CAD build for the part. Positions are in the model's coordinates, mm. A direction names the side the tool comes from. Round coordinates to 2 decimals unless told otherwise and drop trailing zeros. Order: outer loops, then holes, each group sorted by start corner. A loop starts at its lowest first (then second) coordinate and runs counter-clockwise, first axis right, second up. Notation, with made-up numbers: M -13,82.25 L -1,82.25 A14 ccw -1,102.25 Z; hole C 35,17.25 d9. An arc over 180 degrees is marked long. Answer as a JSON object with one key per item and string values.
```python
from build123d import *

# Parameters (mm, degrees)
BOSS_EXTRUDE1_DEPTH       = 138
CUT_EXTRUDE1_DEPTH        = 187.721718073
F_6_0MM_DOWEL_HOLE1_D     = 6
F_6_0MM_DOWEL_HOLE1_DEPTH = 28.197418143
F_6_0MM_DOWEL_HOLE1_TIP   = 1.802581857
M6X1_0_TAPPED_HOLE1_D     = 5
M6X1_0_TAPPED_HOLE1_DEPTH = 21.497848452
M6X1_0_TAPPED_HOLE1_TIP   = 1.502151548
CHAMFER1_SIZE             = 2


with BuildPart() as part:
    # Sketch1 → Boss-Extrude1 (new body)
    with BuildSketch(Plane.XY):
        Polygon((-125, 202.5), (-125, 197.5), (-125, 193), (0, 193), (0, 207), (-125, 207), align=None)
    extrude(amount=BOSS_EXTRUDE1_DEPTH)

    # Sketch3 → Cut-Extrude1 (cut, through all)
    with BuildSketch(Plane(origin=(0, 207, 0), x_dir=(1, 0, 0), z_dir=(0, 1, 0))):
        with BuildLine():
            Line((-105, -30), (-105, -108))
            ThreePointArc((-105, -108), (-102.071067812, -115.071067812), (-95, -118))
            Line((-95, -118), (-30, -118))
            ThreePointArc((-30, -118), (-22.928932188, -115.071067812), (-20, -108))
            Line((-20, -108), (-20, -35.297163281))
            ThreePointArc((-20, -35.297163281), (-18.9403759, -30.817243777), (-15.986064246, -27.286730407))
            ThreePointArc((-15.986064246, -27.286730407), (-14.821532054, -21.896326846), (-20, -20))
            Line((-20, -20), (-95, -20))
            ThreePointArc((-95, -20), (-102.071067812, -22.928932188), (-105, -30))
        make_face()
    extrude(amount=-CUT_EXTRUDE1_DEPTH, mode=Mode.SUBTRACT)

    # Ø6.0mm Dowel Hole1
    with Locations(Plane.XY.offset(20)):
        with Locations((-25, 200), (-55, 200), (-85, 200)):
            Hole(F_6_0MM_DOWEL_HOLE1_D / 2, depth=F_6_0MM_DOWEL_HOLE1_DEPTH)
            with Locations((0, 0, -(F_6_0MM_DOWEL_HOLE1_DEPTH + F_6_0MM_DOWEL_HOLE1_TIP / 2))):  # 118° drill point
                Cone(0, F_6_0MM_DOWEL_HOLE1_D / 2, F_6_0MM_DOWEL_HOLE1_TIP, mode=Mode.SUBTRACT)

    # M6x1.0 Tapped Hole1
    with Locations(Plane.XY.offset(138)):
        with Locations((-95, 200), (-30, 200)):
            Hole(M6X1_0_TAPPED_HOLE1_D / 2, depth=M6X1_0_TAPPED_HOLE1_DEPTH)
            with Locations((0, 0, -(M6X1_0_TAPPED_HOLE1_DEPTH + M6X1_0_TAPPED_HOLE1_TIP / 2))):  # 118° drill point
                Cone(0, M6X1_0_TAPPED_HOLE1_D / 2, M6X1_0_TAPPED_HOLE1_TIP, mode=Mode.SUBTRACT)

    # Chamfer1
    chamfer1_edges = [part.edges().sort_by_distance(p)[0] for p in [
        (0, 193, 69),
        (-125, 193, 69),
        (-18.9403759, 193, 30.817243777),
        (-20, 193, 71.648581641),
        (-22.928932188, 193, 115.071067812),
        (-62.5, 193, 118),
        (-102.071067812, 193, 115.071067812),
        (-105, 193, 69),
        (-102.071067812, 193, 22.928932188),
        (-57.5, 193, 20),
        (-14.821532054, 193, 21.896326846),
    ]]
    chamfer(chamfer1_edges, length=CHAMFER1_SIZE)


solid = part.part
```
Item 1: Wall check: line 1 along X through (y, z) = (200, 127.5); line 2 along X through (y, z) = (200, 12.25); line 3 along X through (y, z) = (195.75, 81). Give the ranges that are in metal, low to high. Write a range as [from, to].
Worked answers:
{"line 1": "x = [-125, -97.5], [-92.5, -32.5], [-27.5, 0]", "line 2": "x = [-125, -88], [-82, -58], [-52, -28], [-22, 0]", "line 3": "x = [-125, -105], [-20, 0]"}
Item 2: Saw through at C-C on z = 125. List the corners of the cut face in (x, y), and give its area (3 significant figures).
Worked answers:
{"outline": "M -125,195 L -123,193 L -2,193 L 0,195 L 0,207 L -125,207 Z; hole C -95,200 d5; hole C -30,200 d5", "area": "1,710 mm2"}
Item 3: 3-axis set-ups, long thin cutter, end or side, ignore diameter. For faces 5 (the conical face through (-102.536, 194.458, 22.628)), 6 (the flat face through (-57, 204, 20)), 7 (the cylindrical face through (-29.67, 202.48, 127.7)), 8 (the cylindrical face through (-55, 203, 10)): which of +Z, -Z, +X, -X, +Y, -Y reach the whole face in a straight line?
Worked answers:
{"face 5": "-Y", "face 6": "+Y, -Y", "face 7": "+Z", "face 8": "-Z"}
Item 4: Saw through at B-B on y = 200. State how many separate pieces and enclosed holes the cut face has, and give its area (3 significant figures).
Worked answers:
{"separate pieces": "5", "enclosed holes": "0", "area": "8,380 mm2"}
Item 5: Saw through at D-D on z = 82. List the corners of the cut face in (x, y), and give its area (3 significant figures).
Worked answers:
{"outline": "M -125,195 L -123,193 L -107,193 L -105,195 L -105,207 L -125,207 Z; M -20,195 L -18,193 L -2,193 L 0,195 L 0,207 L -20,207 Z", "area": "552 mm2"}
Item 6: Saw through at A-A on x = -35. List the corners of the cut face in (y, z), and give its area (3 significant figures).
Worked answers:
{"outline": "M 193,0 L 207,0 L 207,20 L 195,20 L 193,18 Z; M 193,120 L 195,118 L 207,118 L 207,138 L 193,138 Z", "area": "556 mm2"}
Item 7: Two-plate mould, pull along Y, no slides. Class faces 1 (the cylindrical face through (-25, 203, 10)), 2 (the flat face through (-6, 207, 68)), 3 (the cylindrical face through (-14.78, 201.08, 21.97)), 4 (the conical face through (-22.464, 194.458, 115.372)): released by +Y, released by -Y, zero draft, split by the parting line, or undercut.
Worked answers:
{"face 1": "undercut", "face 2": "released by +Y", "face 3": "zero draft", "face 4": "released by -Y"}
